Can you work these out from the drawing? Everything is in mm from the part's minimum corner. A direction names the side the tool comes from. Coordinates: 2 decimals unless noted, no trailing zeros. Order: outer loops, then holes, each group sorted by start corner. A loop starts at its lowest first (then second) coordinate and runs counter-clockwise, first axis right, second up. Notation, with made-up numbers: (1, 32.5) - (42, 32.5) arc R28 ccw to (42, 60.5) - close; hole circle Ø6 at (56.5, 59.5). An arc over 180 degrees is marked (long way). Answer as CSV lines item,"result". Start each with the question number.
Item 1: On a 3-axis mill with a long thin cutter (end or side, diameter ignored), from which of +Z, -Z, +X, -X, +Y, -Y can I reach the whole of each face in a straight line? I mean the marked faces 5 and 6. Say none if no direction works.
Item 2: Imagine slicing it at A-A on z = 30.5. List the corners of the cut face in (x, y) for me (3 decimals).
Item 3: Imagine slicing it at B-B on y = 9. List the corners of the cut face in (x, z) for me (3 decimals).
Item 4: I'm going to push flat-ended pins straight in: pin 1 (6 mm diameter, centred on x = 29, z = 18, fed in from +Y); pin 2 (14 mm diameter, centred on x = 31, z = 12.5, fed in from -Y) (3 decimals); pin 3 (6 mm diameter, centred on x = 16.5, z = 19.5, fed in from +Y); pin 4 (4 mm diameter, centred on x = 23, y = 11.5, fed in from +Z) (3 decimals). Where does each tip first touch, or does it pass through?
Item 5: Imagine slicing it at D-D on z = 15. List the corners of the cut face in (x, y) for me (3 decimals).
Item 6: We'd pull the mould along X, two halves only. Please class the marked faces 1, 2, 3 and 4: pulls with the +X half, pulls with the -X half, needs draft (parallel to the pull), parting line crosses it, or undercut.
Item 7: Imagine slicing it at C-C on x = 29. List the corners of the cut face in (y, z) for me (3 decimals), and give its area (3 significant figures).
Item 8: I need wall thicknesses on line 1 (X direction, y = 21.5, z = 20.5) (3 decimals); line 2 (Z direction, x = 16, y = 43) (3 decimals); line 3 (Y direction, x = 34, z = 10.5) (3 decimals). Which ranges of each line are inside material? Lowest first, please.
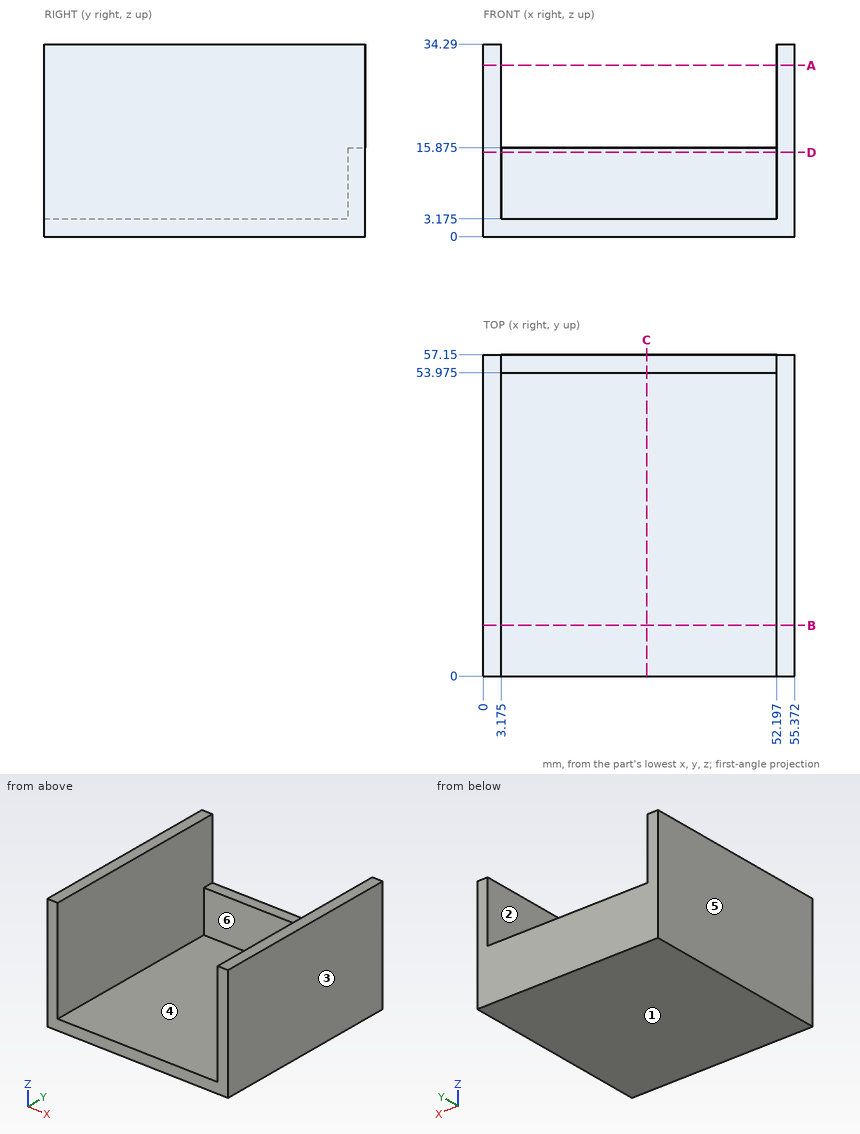
Responses:
1,face 5,"+Z, -Z, -X, +Y, -Y"
1,face 6,"+Z, -Y"
2,outline,"(0, 0) - (3.175, 0) - (3.175, 57.15) - (0, 57.15) - close; (52.197, 0) - (55.372, 0) - (55.372, 57.15) - (52.197, 57.15) - close"
3,outline,"(0, 0) - (55.372, 0) - (55.372, 34.29) - (52.197, 34.29) - (52.197, 3.175) - (3.175, 3.175) - (3.175, 34.29) - (0, 34.29) - close"
4,pin 1,"stops at y = 57.15"
4,pin 2,"stops at y = 53.975"
4,pin 3,"passes through"
4,pin 4,"stops at z = 3.175"
5,outline,"(0, 0) - (3.175, 0) - (3.175, 53.975) - (52.197, 53.975) - (52.197, 0) - (55.372, 0) - (55.372, 57.15) - (0, 57.15) - close"
6,face 1,"needs draft"
6,face 2,"undercut"
6,face 3,"pulls with the +X half"
6,face 4,"undercut"
7,outline,"(0, 0) - (57.15, 0) - (57.15, 15.875) - (53.975, 15.875) - (53.975, 3.175) - (0, 3.175) - close"
7,area,"222 mm^2"
8,line 1,"x = 0 to 3.175, 52.197 to 55.372"
8,line 2,"z = 0 to 3.175"
8,line 3,"y = 53.975 to 57.15"
